Autodesk Inventor part; units mm, degrees
ref_plane "YZ Plane" through (0, 0, 0) normal (1, 0, 0) x (0, 1, 0)
ref_plane "XZ Plane" through (0, 0, 0) normal (0, 1, 0) x (-1, 0, 0)
ref_plane "XY Plane" through (0, 0, 0) normal (0, 0, 1) x (1, 0, 0)
sketch "Эскиз1" plane through (0, 0, 0) normal (0, 0, 1) x (1, 0, 0)
  line L0 (-52.8161, -17.6697) -> (52.3618, -17.6697)
  line L1 (-52.8161, 20.3303) -> (52.3618, 20.3303)
  line L2 (52.3618, 20.3303) -> (52.3618, -17.6697)
  line L3 (52.3618, -17.6697) -> (-52.8161, -17.6697)
  line L4 (-52.8161, -17.6697) -> (-52.8161, 20.3303)
  circle A0 centre (-47.8161, 0.5303) radius 2.1
  circle A1 centre (47.3618, 0.5303) radius 2.1
  point P0 (0, 0)
  point P1 (-8.6177, 20.3303)
extrude "Выдавливание1" add sketch "Эскиз1" along normal blind 3.2
sketch "Эскиз2" plane through (-52.8161, -17.6697, 0) normal (0, -1, 0) x (1, 0, 0)
  line L0 (105.1779, 3.2) -> (0, 3.2)
  line L1 (105.1779, 0) -> (0, 0)
  line L2 (72, 3.2) -> (59, 3.2)
  line L3 (59, 3.2) -> (59, 0)
  line L4 (59, 0) -> (72, 0)
  line L5 (72, 3.2) -> (59, 3.2)
  line L6 (59, 3.2) -> (59, -0.8)
  line L7 (59, -0.8) -> (72, -0.8)
  line L8 (72, -0.8) -> (72, 3.2)
  point P0 (52.8161, 0)
  dimension "d5" = 4
extrude "Выдавливание2" cut sketch "Эскиз2" against normal through all
fillet "Сопряжение1" radius 2 1 edges at (6.1839, 1.3303, 3.2)
sketch "Эскиз3" plane through (-52.8161, -17.6697, 0) normal (0, -1, 0) x (1, 0, 0)
  line L0 (105.1779, 3.2) -> (72, 3.2)
  line L1 (72, 3.2) -> (59, 3.2)
  line L2 (59, 3.2) -> (59, -0.8)
  line L3 (59, -0.8) -> (72, -0.8)
  line L4 (72, -0.8) -> (72, 3.2)
  line L5 (72, -0.8) -> (59, -0.8)
  line L6 (59, -0.8) -> (59, -4)
  line L7 (59, -4) -> (72, -4)
  line L8 (72, -4) -> (72, -0.8)
  line L9 (72, 0) -> (105.1779, 0)
  line L10 (72, -4) -> (75.2, -4)
  line L11 (75.2, -4) -> (75.2, 0)
  line L12 (75.2, 0) -> (72, 0)
  line L13 (72, 0) -> (72, -4)
  line L14 (59, -4) -> (55.8, -4)
  line L15 (55.8, -4) -> (55.8, 0)
  line L16 (55.8, 0) -> (59, 0)
  line L17 (59, 0) -> (59, -4)
  point P0 (52.8161, 0)
  dimension "d6" = 13
  dimension "d7" = 4
  dimension "d8" = 13
  dimension "d9" = 3.2
  dimension "d10" = 3.2
  dimension "d11" = 3.2
extrude "Выдавливание3" add sketch "Эскиз3" against normal up to surface (38 mm away) contours L9 L11 L10 L8 L4 | L2 L6 L14 L15 L16 | L8 L7 L6 L3
fillet "Сопряжение2" radius 2 1 edges at (19.1839, 1.3303, 3.2)
fillet "Сопряжение3" radius 9 2 edges at (22.3839, 1.3303, 0) (2.9839, 1.3303, 0)
fillet "Сопряжение4" radius 3.25 2 edges at (2.9839, 1.3303, -4) (22.3839, 1.3303, -4)
sketch "Эскиз4" plane through (0, 0, 0) normal (0, 0, -1) x (-1, 0, 0)
  line L0 (30.891, 20.3303) -> (19.391, 20.3303)
  line L1 (30.891, -17.6697) -> (30.891, 20.3303)
  line L2 (19.391, -17.6697) -> (30.891, -17.6697)
  line L3 (19.391, -17.6697) -> (19.391, 20.3303)
  circle A0 centre (24.991, 0.5303) radius 2.1
  line L4 (4.4994, -17.6697) -> (4.4994, 20.3303)
  line L5 (52.8161, -17.6697) -> (4.4994, -17.6697)
  line L6 (52.8161, 20.3303) -> (52.8161, -17.6697)
  line L7 (4.4994, 20.3303) -> (52.8161, 20.3303)
  circle A1 centre (47.8161, 0.5303) radius 2.1
  point P0 (0, 0)
extrude "Выдавливание4" cut sketch "Эскиз4" against normal blind 10 contours L7 L6 L5 L1 | A0
properties part number "драйвер 2"
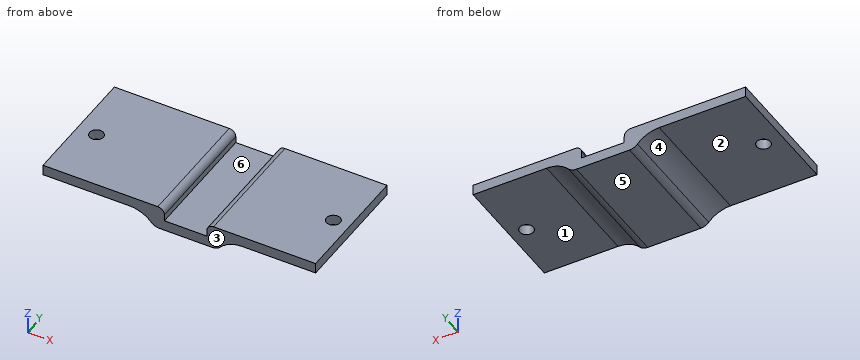
Could you check a few things on this model? Use its own coordinates, in mm. Face numbers are marked on the shaded views. A direction names the side the tool comes from. Give positions to 0.01 mm unless a question says otherwise; leave off trailing zeros. Order: outer loops, then holes, each group sorted by start corner. A loop starts at its lowest first (then second) coordinate and runs counter-clockwise, first axis right, second up.
Q1. Suppose I cut it at B-B, the plane x = -19. Write out the boundary of the cut face in (y, z), and give its area (3 significant figures).
Q2. I'm going to push flat-ended pins straight in: P1, Ø21, axis at x = -11.5, y = 10.5, coming from the -Z side; P2, Ø5.5, axis at x = -24.99, y = 0.53, coming from the -Z side; P3, Ø6.5, axis at x = 12.5, y = 1.5, coming from the +Z side. Where does each tip first touch, or does it pass through?
Q3. Suppose I cut it at A-A, the plane y = -8. Write out the boundary of the cut face in (x, z), and give its area (3 significant figures).
Q4. If I drill on line 1 along X through (y, z) = (13.5, 0.5); line 2 along Z through (x, y) = (11, -16); line 3 along Z through (x, y) = (-5.5, 1.5), over which ranges is the centre line in solid material (lowest first)?
Q5. For the marked faces 1, 2 and 3, which set-ups out of +Z, -Z, +X, -X, +Y, -Y let a thin tool reach every point of the face, with its end or its side?
Q6. Suppose I cut it at C-C, the plane x = 3. Write out the boundary of the cut face in (y, z), and give its area (3 significant figures).
Q7. We'd pull the mould along X, two halves only. Please class the marked faces 4, 5 and 6: +X half, -X half, draft (parallel to the pull), parting line (faces both ways), or undercut.
Solution:
1. outline: (-17.67, 0) - (20.33, 0) - (20.33, 3.2) - (-17.67, 3.2) - close
1. area: 122 mm2
2. P1: stops at z = -0.71
2. P2: stops at z = 0
2. P3: stops at z = -0.8
3. outline: (-30.89, 0) - (-4.5, 0) arc R9 cw to (2.15, -2.94) arc R3.25 ccw to (4.56, -4) - (20.81, -4) arc R3.25 ccw to (23.21, -2.94) arc R9 cw to (29.87, 0) - (52.36, 0) - (52.36, 3.2) - (21.18, 3.2) arc R2 ccw to (19.18, 1.2) - (19.18, -0.8) - (6.18, -0.8) - (6.18, 1.2) arc R2 ccw to (4.18, 3.2) - (-30.89, 3.2) - close
3. area: 307 mm2
4. line 1: x = -30.89 to 6.18, 19.18 to 52.36
4. line 2: z = -4 to -0.8
4. line 3: z = 0 to 3.2
5. face 1: -Z, +X, +Y, -Y
5. face 2: -Z, -X, +Y, -Y
5. face 3: +Z, -Z, +X, -X, -Y
6. outline: (-17.67, -3.6) - (20.33, -3.6) - (20.33, 3.2) - (-17.67, 3.2) - close
6. area: 259 mm2
7. face 4: -X half
7. face 5: draft
7. face 6: undercut
